```python
from build123d import *

# Parameters (mm, degrees)
SKETCH_1_R      = 135
SKETCH_1_R_2    = 50
EXTRUDE_1_DEPTH = 80
FILLET_4_R      = 20
FILLET_5_R      = 20
FILLET_6_R      = 35
FILLET_7_R      = 35


with BuildPart() as part:
    # Эскиз1 → Вытянуть1 (new body)
    with BuildSketch(Plane.XY):
        Circle(SKETCH_1_R)
        Circle(SKETCH_1_R_2, mode=Mode.SUBTRACT)
    extrude(amount=EXTRUDE_1_DEPTH)

    # Скругление4
    fillet_4_edges = [part.edges().sort_by_distance(p)[0] for p in [
        (-135, 0, 0),
    ]]
    fillet(fillet_4_edges, radius=FILLET_4_R)

    # Скругление5
    fillet_5_edges = [part.edges().sort_by_distance(p)[0] for p in [
        (-135, 0, 80),
    ]]
    fillet(fillet_5_edges, radius=FILLET_5_R)

    # Скругление6
    fillet_6_edges = [part.edges().sort_by_distance(p)[0] for p in [
        (-50, 0, 0),
    ]]
    fillet(fillet_6_edges, radius=FILLET_6_R)

    # Скругление7
    fillet_7_edges = [part.edges().sort_by_distance(p)[0] for p in [
        (-50, 0, 80),
    ]]
    fillet(fillet_7_edges, radius=FILLET_7_R)


solid = part.part
```
The listing builds one solid part. Answer for the finished solid, in the listing's coordinates (mm). Coordinates: 2 decimals unless noted, no trailing zeros. Loops run counter-clockwise (first coordinate to the right, second up) from the corner with the lowest first, then second, coordinate; pieces in that order, holes last. Notation, with made-up numbers: M 42.25,43.25 L 80.25,43.25 A29 cw 80.25,77.25 Z; hole C -6.5,28.25 d3. An arc over 180 degrees is marked long. Answer as a JSON object with one key per item and string values. Group by question number.
Item 1: Consider L1, parallel to Y at x = 0, z = 40; L2, parallel to Y at x = 5.5, z = 37.5; L3, parallel to Z at x = 17, y = -115.5. Determine where each line is inside the solid, lowest interval first.
Item 2: Section A-A (x = 0) is taken. Write down the section's boundary in (y, z), and give its area (3 significant figures).
Item 3: Each of these flat-tipped pins is pushed along its axis until it touches: P1, Ø8, axis at x = 48.5, y = 6, coming from the -Z side; P2, Ø1, axis at x = 86, z = 15.5, coming from the -Y side; P3, Ø1.5, axis at x = 102.5, z = 46, coming from the -Y side. Where does it stop, or does it pass through?
Item 4: Section D-D (z = 55) is taken. Write down the section's boundary in (x, y).
Item 5: Section C-C (z = 16) is taken. Write down the section's boundary in (x, y), and give its area (3 significant figures).
Solved:
{
 "1": {"L1": "y = -135 to -50, 50 to 135", "L2": "y = -134.89 to -49.7, 49.7 to 134.89", "L3": "z = 0.08 to 79.92"},
 "2": {"outline": "M -135,20 A20 ccw -115,0 L -85,0 A35 ccw -50,35 L -50,45 A35 ccw -85,80 L -115,80 A20 ccw -135,60 Z; M 50,35 A35 ccw 85,0 L 115,0 A20 ccw 135,20 L 135,60 A20 ccw 115,80 L 85,80 A35 ccw 50,45 Z", "area": "12,200 mm2"},
 "3": {"P1": "stops at z = 21.12", "P2": "stops at y = -103.84", "P3": "stops at y = -88.72"},
 "4": {"outline": "C 0,0 d270; hole C 0,0 d102.92"},
 "5": {"outline": "C 0,0 d269.19; hole C 0,0 d111.21", "area": "47,200 mm2"}
}
